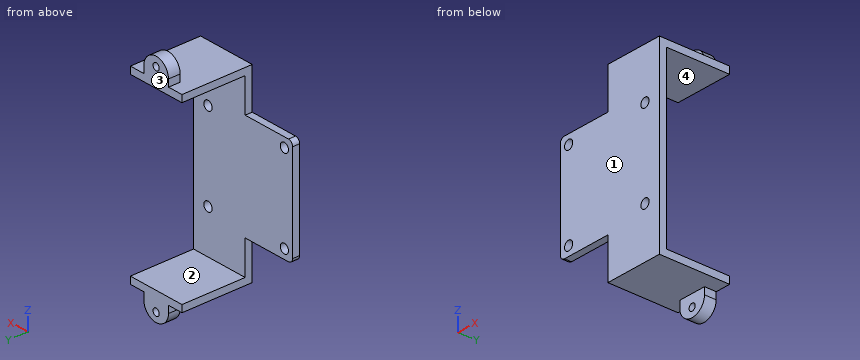
```python
from build123d import *

# Parameters (mm, degrees)
EXTRUDE_1_OUTLINE_W = 25
EXTRUDE_1_OUTLINE_H = 80
EXTRUDE_1_DEPTH     = 30
SKETCH_2_W          = 74
SKETCH_2_H          = 27
CUT_EXTRUDE_1_DEPTH = 33
SKETCH_3_R          = 1.5
EXTRUDE_2_DEPTH     = 5
SKETCH_4_R          = 2
EXTRUDE_3_DEPTH     = 3
SKETCH_5_R          = 2
CUT_EXTRUDE_2_DEPTH = 3


# Read off the part's stored shape, not the designer's step: 填料-伸長1
with BuildPart() as part:
    # 填料-伸長1 outline → 填料-伸長1 (new body)
    with BuildSketch(Plane.XZ.offset(-131.641882403)):
        with Locations((29.792094012, -19.915289206)):
            Rectangle(EXTRUDE_1_OUTLINE_W, EXTRUDE_1_OUTLINE_H)
    extrude(amount=EXTRUDE_1_DEPTH)

    # 草圖2 → 除料-伸長1 (cut)
    with BuildSketch(Plane(origin=(42.292094012, 0, 0), x_dir=(0, 0, -1), z_dir=(1, 0, 0))):
        with Locations((19.915289206, 118.141882403)):
            Rectangle(SKETCH_2_W, SKETCH_2_H)
    extrude(amount=-CUT_EXTRUDE_1_DEPTH, mode=Mode.SUBTRACT)

    # 草圖3 → 填料-伸長2 (add)
    # profile 1 of 2: a face of its own
    with BuildSketch(Plane.XZ.offset(-131.641882403)):
        with BuildLine():
            Line((23.792094012, 20.084710794), (35.792094012, 20.084710794))
            Line((35.792094012, 20.084710794), (35.792094012, 23.084710794))
            ThreePointArc((35.792094012, 23.084710794), (29.792094012, 28.938496633), (23.792094012, 23.084710794))
            Line((23.792094012, 23.084710794), (23.792094012, 20.084710794))
        make_face()
        with Locations(Location((29.792094012, 25.084710794, 0), (0, 0, 270))):
            Circle(SKETCH_3_R, mode=Mode.SUBTRACT)
    # profile 2 of 2: a face of its own
    with BuildSketch(Plane.XZ.offset(-131.641882403)):
        with BuildLine():
            Line((23.792094012, -62.915289206), (23.792094012, -59.915289206))
            Line((23.792094012, -59.915289206), (35.792094012, -59.915289206))
            Line((35.792094012, -59.915289206), (35.792094012, -62.915289206))
            ThreePointArc((35.792094012, -62.915289206), (29.792094012, -68.769075045), (23.792094012, -62.915289206))
        make_face()
        with Locations(Location((29.792094012, -64.915289206, 0), (0, 0, 90))):
            Circle(SKETCH_3_R, mode=Mode.SUBTRACT)
    extrude(amount=EXTRUDE_2_DEPTH)

    # 草圖4 → 填料-伸長3 (add)
    with BuildSketch(Plane.XZ.offset(-101.641882403)):
        with BuildLine():
            Line((17.292094012, 2.584710794), (-3.707905988, 2.584710794))
            ThreePointArc((-3.707905988, 2.584710794), (-5.12211955, 1.998924356), (-5.707905988, 0.584710794))
            Line((-5.707905988, 0.584710794), (-5.707905988, -40.415289206))
            ThreePointArc((-5.707905988, -40.415289206), (-5.12211955, -41.829502769), (-3.707905988, -42.415289206))
            Line((-3.707905988, -42.415289206), (17.292094012, -42.415289206))
            Line((17.292094012, -42.415289206), (17.292094012, 2.584710794))
        make_face()
        with Locations(Location((-1.707905988, -38.415289206, 0), (0, 0, 270))):
            Circle(SKETCH_4_R, mode=Mode.SUBTRACT)
        with Locations(Location((-1.707905988, -1.415289206, 0), (0, 0, 270))):
            Circle(SKETCH_4_R, mode=Mode.SUBTRACT)
    extrude(amount=-EXTRUDE_3_DEPTH)

    # 草圖5 → 除料-伸長2 (cut)
    with BuildSketch(Plane.XZ.offset(-101.641882403)):
        with Locations(Location((35.292094012, -1.415289206, 0), (0, 0, 270))):
            Circle(SKETCH_5_R)
        with Locations(Location((35.292094012, -38.415289206, 0), (0, 0, 270))):
            Circle(SKETCH_5_R)
    extrude(amount=-CUT_EXTRUDE_2_DEPTH, mode=Mode.SUBTRACT)


solid = part.part
```
Part model, mm, in its own coordinate system. Face numbers are marked on the shaded views. A direction names the side the tool comes from. Give positions to 0.01 mm unless a question says otherwise; leave off trailing zeros. Order: outer loops, then holes, each group sorted by start corner. A loop starts at its lowest first (then second) coordinate and runs counter-clockwise, first axis right, second up. Notation, with made-up numbers: M 24.5,20 L 82.5,20 A15 ccw 82.5,45 Z; hole C 55,-20.75 d10. An arc over 180 degrees is marked long. Use a Markdown table: item, result. Add a question column.
(1) 3-axis set-ups, long thin cutter, end or side, ignore diameter. For the marked faces 3 and 4: which of +Z, -Z, +X, -X, +Y, -Y reach the whole face in a straight line?
(2) Drop flat-ended pins along their axis: P1, Ø2.5, axis at x = 7.5, y = 103, coming from the -Z side; P2, Ø12, axis at x = 25, y = 107.5, coming from the -Z side; P3, Ø24, axis at x = 27, z = -2, coming from the +Y side. Give the stop position or say it passes through.
(3) Saw through at D-D, the plane z = -38. Give the cut face in (x, y).
(4) Saw through at C-C, the plane x = 22.5. Give the cut face in (y, z), and give its area (3 significant figures).
(5) Probe line 1 along Z through (x, y) = (28.5, 125); line 2 along Z through (x, y) = (-1, 103); line 3 along Y through (x, z) = (18, -19.5). List the from-to ranges inside material, lowest first. Write a range as [from, to].
(6) Mould opens along Z. For the marked faces 1 and 2 say: +Z half, -Z half, draft (parallel to the pull), parting line (faces both ways), or undercut.
(7) Saw through at B-B, the plane y = 111. Give the cut face in (x, z).
Answer key:
| question | item | result |
|---|---|---|
| 1 | face 3 | +Z, -Z, +X, -X, +Y |
| 1 | face 4 | +X, -X, +Y |
| 2 | P1 | z = -42.42 |
| 2 | P2 | z = -59.92 |
| 2 | P3 | y = 104.64 |
| 3 | outline | M -5.71,101.64 L -3.66,101.64 L -3.66,104.64 L -5.71,104.64 Z; M 0.25,101.64 L 33.34,101.64 L 33.34,104.64 L 0.25,104.64 Z; M 37.25,101.64 L 42.29,101.64 L 42.29,104.64 L 37.25,104.64 Z |
| 4 | outline | M 101.64,-59.92 L 131.64,-59.92 L 131.64,-56.92 L 104.64,-56.92 L 104.64,17.08 L 131.64,17.08 L 131.64,20.08 L 101.64,20.08 Z |
| 4 | area | 402 mm^2 |
| 5 | line 1 | [-59.92, -56.92], [17.08, 20.08] |
| 5 | line 2 | [-42.42, -40.29], [-36.54, -3.29], [0.46, 2.58] |
| 5 | line 3 | [101.64, 104.64] |
| 6 | face 1 | draft |
| 6 | face 2 | undercut |
| 7 | outline | M 17.29,-59.92 L 42.29,-59.92 L 42.29,-56.92 L 17.29,-56.92 Z; M 17.29,17.08 L 42.29,17.08 L 42.29,20.08 L 17.29,20.08 Z |
